from build123d import *

# Parameters (mm, degrees)
SKETCH1_R           = 2.5
BOSS_EXTRUDE1_DEPTH = 5
SKETCH2_R           = 2.5
CUT_EXTRUDE1_DEPTH  = 9
CIRPATTERN1_COUNT   = 6


with BuildPart() as part:
    # Sketch1 → Boss-Extrude1 (new body)
    with BuildSketch(Plane.XY):
        Polygon((-8.789542733, 5.544721683), (-9.196641201, -4.839606453), (-0.407098468, -10.384328136), (8.789542733, -5.544721683), (9.196641201, 4.839606453), (0.407098468, 10.384328136), align=None)
        Circle(SKETCH1_R, mode=Mode.SUBTRACT)
    extrude(amount=BOSS_EXTRUDE1_DEPTH)

    # Sketch2 → Cut-Extrude1 (cut)
    with BuildSketch(Plane.XY.offset(5)):
        with Locations((-2.677725251, 5.08844647)):
            Circle(SKETCH2_R)
    cut_extrude1 = extrude(amount=-CUT_EXTRUDE1_DEPTH, mode=Mode.SUBTRACT)

    # CirPattern1: Cut-Extrude1 ×6 about axis
    cirpattern1_axis = Axis((0, 0, 0), (0, 0, 1))
    for i in range(1, CIRPATTERN1_COUNT):
        add(cut_extrude1.rotate(cirpattern1_axis, i * 360 / CIRPATTERN1_COUNT), mode=Mode.SUBTRACT)


solid = part.part
The model under review builds one solid part; all positions refer to its coordinate system, in mm. Give positions to 0.01 mm unless a question says otherwise; leave off trailing zeros. Order: outer loops, then holes, each group sorted by start corner. A loop starts at its lowest first (then second) coordinate and runs counter-clockwise, first axis right, second up. Notation, with made-up numbers: M -34.5,40 L 16.5,40 A12 ccw 16.5,62 Z; hole C 25,43 d5. An arc over 180 degrees is marked long. Use one line per item in the form item = value. Start each with the question number.
Item 1: We need section D-D on x = 4. Give the boundary of the cut face in (y, z).
Item 2: To check wall thickness, follow line 1 along X through (y, z) = (4, 4.5); line 2 along X through (y, z) = (3, 3.8); line 3 along X through (y, z) = (-1.25, 1.6). State the ranges of each line that lie inside material, in increasing order. Write a range as from..to.
Item 3: We need section C-C on y = 0. Give the boundary of the cut face in (x, z).
Item 4: Insertion check: pin 1 Ø3 at (y, z) = (2.5, 2.5) entering from +X; pin 2 Ø1 at (y, z) = (1.5, 2) entering from -X; pin 3 Ø3 at (x, z) = (2, 2.5) entering from -Y. Each pin has a flat end and moves straight along its axis. Give the tip position at first contact, or say it passes through.
Item 5: We need section B-B on x = 7.5. Give the boundary of the cut face in (y, z), plus the area to 3 significant figures.
Item 6: We need section A-A on y = -6. Give the boundary of the cut face in (x, z).
Item 7: The part is to be moulded in two halves that separate along X. For faces 1 (the cylindrical face through (4.91, 3.174, 2.535)), 2 (the flat face through (2, -2, 5)), 3 (the flat face through (-8.99, 0.43, 2.46)), 4 (the flat face through (4.863, 7.573, 2.465)), say which applies: pulls with the +X half, pulls with the -X half, needs draft (parallel to the pull), parting line crosses it, or undercut.
Completed:
q1.outline = M -8.07,0 L -7.21,0 L -7.21,5 L -8.07,5 Z; M -2.97,0 L -2.01,0 L -2.01,5 L -2.97,5 Z; M 1.56,0 L 2.54,0 L 2.54,5 L 1.56,5 Z; M 7.18,0 L 8.12,0 L 8.12,5 L 7.18,5 Z
q2.line_1 = -8.85..-4.93, -0.43..0.72, 5.41..9.16
q2.line_2 = -8.89..-4.05, -1.3..1.4, 4.73..9.12
q2.line_3 = -9.06..-7.76, -3.73..-2.17, 2.17..3.47, 8.03..8.96
q3.outline = M -9.01,0 L -8.24,0 L -8.24,5 L -9.01,5 Z; M -3.26,0 L -2.5,0 L -2.5,5 L -3.26,5 Z; M 2.5,0 L 3.26,0 L 3.26,5 L 2.5,5 Z; M 8.24,0 L 9.01,0 L 9.01,5 L 8.24,5 Z
q4.pin_1 = 9.16
q4.pin_2 = -8.97
q4.pin_3 = -9.91
q5.outline = M -6.22,0 L -2.01,0 L -2.01,5 L -6.22,5 Z; M 1.56,0 L 5.91,0 L 5.91,5 L 1.56,5 Z
q5.area = 42.9 mm²
q6.outline = M -7.36,0 L -5.29,0 L -5.29,5 L -7.36,5 Z; M -0.84,0 L 0.35,0 L 0.35,5 L -0.84,5 Z; M 5.01,0 L 7.92,0 L 7.92,5 L 5.01,5 Z
q7.face_1 = undercut
q7.face_2 = needs draft
q7.face_3 = pulls with the -X half
q7.face_4 = pulls with the +X half
